from build123d import *

# Parameters (mm, degrees)
F0_W           = 25
F0_H           = 52
F1_DEPTH       = 3
F2_R           = 5
F4_D           = 4
F4_CSINK_D     = 6.5
F4_CSINK_ANGLE = 90
F5_D           = 21


with BuildPart() as f1:
    # F0 (on Front) → F1 (new body)
    with BuildSketch(Plane.XZ):
        with Locations((12.5, 26)):
            Rectangle(F0_W, F0_H)
    extrude(amount=F1_DEPTH)

    # F2
    f2_edges = [f1.edges().sort_by_distance(p)[0] for p in [
        (25, -1.5, 52),
        (0, -1.5, 52),
        (0, -1.5, 0),
        (25, -1.5, 0),
    ]]
    fillet(f2_edges, radius=F2_R)

    # F4 (through all)
    with Locations(Plane.XZ.offset(3)):
        with Locations((12.5, 47), (12.5, 5)):
            CounterSinkHole(F4_D / 2, F4_CSINK_D / 2, counter_sink_angle=F4_CSINK_ANGLE)

    # F5 (through all)
    with Locations(Plane.XZ.offset(3)):
        with Locations((12.5, 26)):
            Hole(F5_D / 2)


solid = f1.part
Verification items for the finished model (mm, model axes). Give positions to 0.01 mm unless a question says otherwise; leave off trailing zeros. Loops run counter-clockwise (first coordinate to the right, second up) from the corner with the lowest first, then second, coordinate; pieces in that order, holes last. Notation, with made-up numbers: (81.5, -38) - (88.5, -38) arc R21 cw to (88.5, -12) - close; hole circle Ø8 at (-14.75, 4). An arc over 180 degrees is marked (long way). Write item = value, one per line. Start each with the question number.
Q1. Cross-section at A-A, the plane x = 12.5. Enter the section's corners in (y, z).
Q2. Cross-section at D-D, the plane x = 4. Enter the section's corners in (y, z).
Q3. Depth check by flat-ended pin: P1, Ø5, axis at x = 12.5, z = 5, coming from the -Y side. Enter the tip coordinate at first touch or a pass-through.
Q4. Cross-section at C-C, the plane z = 28. Enter the section's corners in (x, y).
Q5. Cross-section at B-B, the plane y = -0.7. Enter the section's corners in (x, z).
Q6. Thickness scan on line 1 (Z direction, x = 12.5, y = -0.6); line 2 (X direction, y = -0.35, z = 47); line 3 (Z direction, x = 11.5, y = -2.3). Record the ranges inside material, lowest first.
Q7. Mould release check, pull along Z, two halves, no side actions. Record for faces 1 (the face through (25, -1, 26)), 2 (the face through (12, -1, 52)), 3 (the face through (14.498, -0.863, 5.088)): released by +Z, released by -Z, zero draft, split by the parting line, or undercut.
Answer key:
q1.outline = (-3, 0) - (0, 0) - (0, 3) - (-1.75, 3) - (-3, 1.75) - close; (-3, 8.25) - (-1.75, 7) - (0, 7) - (0, 15.5) - (-3, 15.5) - close; (-3, 36.5) - (0, 36.5) - (0, 45) - (-1.75, 45) - (-3, 43.75) - close; (-3, 50.25) - (-1.75, 49) - (0, 49) - (0, 52) - (-3, 52) - close
q2.outline = (-3, 0.1) - (0, 0.1) - (0, 19.84) - (-3, 19.84) - close; (-3, 32.16) - (0, 32.16) - (0, 51.9) - (-3, 51.9) - close
q3.P1 = -2.25
q4.outline = (0, -3) - (2.19, -3) - (2.19, 0) - (0, 0) - close; (22.81, -3) - (25, -3) - (25, 0) - (22.81, 0) - close
q5.outline = (0, 5) arc R5 ccw to (5, 0) - (20, 0) arc R5 ccw to (25, 5) - (25, 47) arc R5 ccw to (20, 52) - (5, 52) arc R5 ccw to (0, 47) - close; hole circle Ø21 at (12.5, 26); hole circle Ø4 at (12.5, 5); hole circle Ø4 at (12.5, 47)
q6.line_1 = 0 to 3, 7 to 15.5, 36.5 to 45, 49 to 52
q6.line_2 = 0 to 10.5, 14.5 to 25
q6.line_3 = 0 to 2.65, 7.35 to 15.55, 36.45 to 44.65, 49.35 to 52
q7.face_1 = zero draft
q7.face_2 = released by +Z
q7.face_3 = undercut
